CAD build for the part. Positions are in the model's coordinates, mm. A direction names the side the tool comes from. Coordinates: 2 decimals unless noted, no trailing zeros. Loops run counter-clockwise (first coordinate to the right, second up) from the corner with the lowest first, then second, coordinate; pieces in that order, holes last. Notation, with made-up numbers: (75, 22.25) -> (84, 22.25) arc R18 ccw to (84, 39.25) -> close; hole circle Ø6 at (87, 81). An arc over 180 degrees is marked (long way). Write each question's results on one line, items separated by ' | '.
Autodesk Inventor part; units mm, degrees
ref_plane "Work Plane1" through (-17, 0, 36) normal (0.7071, 0, 0.7071) x (0.7071, 0, -0.7071)
ref_plane "YZ Plane" through (0, 0, 0) normal (1, 0, 0) x (0, 1, 0)
ref_plane "XY Plane" through (0, 0, 0) normal (0, 0, 1) x (1, 0, 0)
sketch "Sketch1" plane through (0, 0, 0) normal (0, 0, 1) x (1, 0, 0)
  circle A0 centre (0, 0) radius 17
  dimension "d0" = 34
extrude "Extrusion1" add sketch "Sketch1" along normal blind 36
sketch "Sketch2" plane through (0, 0, 0) normal (0, 1, 0) x (-1, 0, 0)
  line L0 (17, 36) -> (-17, 36)
  line L1 (17, 36) -> (-17.212, 1.788)
  point P0 (0, 0)
  dimension "d3" = 45
ref_plane "Work Plane1" through (-17, 0, 36) normal (0.7071, 0, 0.7071) x (0.7071, 0, -0.7071)
split "Split2" plane through (-17, 0, 36) removes the side toward (0.7071, 0, 0.7071)
sketch "Sketch3" plane through (0, 0, 0) normal (0, 0, -1) x (-1, 0, 0)
  circle A0 centre (0, 0) radius 12
  circle A1 centre (6.0165, -10.3828) radius 2.5
  circle A2 centre (5.9835, 10.4018) radius 2.5
  circle A3 centre (-12, -0.0191) radius 2.5
  dimension "d5" = 24
  dimension "d6" = 5
  dimension "d9" = 360
extrude "Extrusion2" cut sketch "Sketch3" against normal blind 3 contours A2 A0 | A0 A2 | A1 A0 | A0 A1 | A3 A0 | A0 A3
sketch "Sketch4" plane through (0, 0, 0) normal (0, 0, -1) x (-1, 0, 0)
  point P0 (0, -12)
properties part number "trzymadlo" material "ABS Plastic"
1) Pin check, flat tips, straight feed: pin 1 (4 mm diameter, centred on x = -6.02, y = -10.38, fed in from +Z); pin 2 (6 mm diameter, centred on x = -11, z = 4, fed in from +Y); pin 3 (4 mm diameter, centred on y = -7.5, z = 31, fed in from +X). Stop position of each tip, or through.
Outcome:
pin 1: stops at z = 27.02 | pin 2: stops at y = 15 | pin 3: stops at x = -10
2) Which spindle directions (+Z, -Z, +X, -X, +Y, -Y) get a long thin tool onto all of the face, cutting with end or side? Do faces 4 (the cylindrical face through (-16.984, -0.747, 13.748)), 5 (the flat face through (-6, -10, 3)). Say none if no direction does.
Outcome:
face 4: +Z, -Z | face 5: -Z
3) Two-plate mould, pull along X, no slides. Class faces 1 (the cylindrical face through (-8.326, -11.34, 1.479)), 2 (the flat face through (0, 0, 0)), 3 (the flat face through (0, 0, 19)): pulls with the +X half, pulls with the -X half, needs draft (parallel to the pull), parting line crosses it, or undercut.
Outcome:
face 1: undercut | face 2: needs draft | face 3: pulls with the +X half
4) Drill centre lines: L1, parallel to Y at x = 12, z = 1.85; L2, parallel to Y at x = 0.5, z = 17.5; L3, parallel to Y at x = -14.5, z = 12. Where is each one in solid material? Low to high. Write a range as from..to.
Outcome:
L1: y = -12.04..-2.52, 2.48..12.04 | L2: y = -16.99..16.99 | L3: y = -8.87..8.87
5) Slice it at D-D (x = 0). Write the cut outline in (y, z), then the cut area to 3 significant figures.
Outcome:
outline: (-17, 0) -> (17, 0) -> (17, 19) -> (-17, 19) -> close | area: 646 mm^2
6) Slice it at B-B (y = 1). Write the cut outline in (x, z), then the cut area to 3 significant figures.
Outcome:
outline: (-16.97, 0) -> (9.72, 0) -> (9.72, 3) -> (14.28, 3) -> (14.28, 0) -> (16.97, 0) -> (16.97, 2.03) -> (-16.97, 35.97) -> close | area: 631 mm^2
7) Slice it at C-C (z = 11). Write the cut outline in (x, y), then the cut area to 3 significant figures.
Outcome:
outline: (8, -15) -> (8, 15) arc R17 ccw (long way) to start | area: 716 mm^2
8) Slice it at A-A (x = 10). Write the cut outline in (y, z), then the cut area to 3 significant figures.
Outcome:
outline: (-13.75, 0) -> (-1.52, 0) -> (-1.52, 3) -> (1.48, 3) -> (1.48, 0) -> (13.75, 0) -> (13.75, 9) -> (-13.75, 9) -> close | area: 238 mm^2
